from build123d import *

# Parameters (mm, degrees)
CROQUIS1_W              = 164.9
CROQUIS1_H              = 102
SALIENTE_EXTRUIR2_DEPTH = 14.27
CROQUIS2_W              = 174.9
CROQUIS2_H              = 112
CROQUIS2_W_2            = 166.9
CROQUIS2_H_2            = 104
SALIENTE_EXTRUIR3_DEPTH = 14.27
CROQUIS3_W              = 174.9
CROQUIS3_H              = 112
CROQUIS3_W_2            = 160.9
CROQUIS3_H_2            = 98.374406292
SALIENTE_EXTRUIR5_DEPTH = 1
CROQUIS4_W              = 164.9
CROQUIS4_H              = 102
CORTAR_EXTRUIR2_DEPTH   = 14.27
CROQUIS6_W              = 174.9
CROQUIS6_H              = 112
CROQUIS6_R              = 1.5
SALIENTE_EXTRUIR6_DEPTH = 15
CROQUIS8_W              = 160.9
CROQUIS8_H              = 98.374406292
CORTAR_EXTRUIR3_DEPTH   = 9
CROQUIS9_W              = 166.9
CROQUIS9_H              = 104
CORTAR_EXTRUIR5_DEPTH   = 11
CROQUIS15_W             = 6.3
CROQUIS15_H             = 15
CROQUIS15_W_2           = 3.5
CROQUIS15_H_2           = 7
CORTAR_EXTRUIR6_DEPTH   = 7
CORTAR_EXTRUIR7_DEPTH   = 7
CROQUIS17_R             = 4
CORTAR_EXTRUIR8_DEPTH   = 7
CROQUIS18_W             = 4
CROQUIS18_H             = 16
CORTAR_EXTRUIR9_DEPTH   = 7
CROQUIS21_R             = 1.5
CORTAR_EXTRUIR12_DEPTH  = 25.4
CROQUIS22_W             = 4.034105038
CROQUIS22_H             = 112
CORTAR_EXTRUIR13_DEPTH  = 179.4


with BuildPart() as part:
    # Croquis1 → Saliente-Extruir2 (new body)
    with BuildSketch(Plane(origin=(0, 0, 0), x_dir=(0, 0, -1), z_dir=(1, 0, 0))):
        Rectangle(CROQUIS1_W, CROQUIS1_H)
    extrude(amount=SALIENTE_EXTRUIR2_DEPTH)

    # Croquis4 → Cortar-Extruir2 (cut)
    with BuildSketch(Plane(origin=(14.27, 0, 0), x_dir=(0, 0, -1), z_dir=(1, 0, 0))):
        Rectangle(CROQUIS4_W, CROQUIS4_H)
    extrude(amount=-CORTAR_EXTRUIR2_DEPTH, mode=Mode.SUBTRACT)


with BuildPart() as body_2:
    # Croquis2 → Saliente-Extruir3 (new body)
    with BuildSketch(Plane(origin=(0, 0, 0), x_dir=(0, 0, -1), z_dir=(1, 0, 0))):
        Rectangle(CROQUIS2_W, CROQUIS2_H)
        Rectangle(CROQUIS2_W_2, CROQUIS2_H_2, mode=Mode.SUBTRACT)
    extrude(amount=SALIENTE_EXTRUIR3_DEPTH)

    # Croquis3 → Saliente-Extruir5 (add)
    with BuildSketch(Plane.ZY):
        Rectangle(CROQUIS3_W, CROQUIS3_H)
        with Locations((0, -0.062203146)):
            Rectangle(CROQUIS3_W_2, CROQUIS3_H_2, mode=Mode.SUBTRACT)
    extrude(amount=SALIENTE_EXTRUIR5_DEPTH)

    # Croquis6 → Saliente-Extruir6 (add)
    with BuildSketch(Plane(origin=(14.27, 0, 0), x_dir=(0, 0, -1), z_dir=(1, 0, 0))):
        Rectangle(CROQUIS6_W, CROQUIS6_H)
        with Locations((-77.445, 46)):
            Circle(CROQUIS6_R, mode=Mode.SUBTRACT)
        with Locations((-77.445, -46)):
            Circle(CROQUIS6_R, mode=Mode.SUBTRACT)
        with Locations((-22.1, 15.81)):
            Circle(CROQUIS6_R, mode=Mode.SUBTRACT)
        with Locations((35.9, 15.81)):
            Circle(CROQUIS6_R, mode=Mode.SUBTRACT)
        with Locations((-22.1, -33.19)):
            Circle(CROQUIS6_R, mode=Mode.SUBTRACT)
        with Locations((35.9, -33.19)):
            Circle(CROQUIS6_R, mode=Mode.SUBTRACT)
        with Locations((77.445, 46)):
            Circle(CROQUIS6_R, mode=Mode.SUBTRACT)
        with Locations((77.445, -46)):
            Circle(CROQUIS6_R, mode=Mode.SUBTRACT)
    extrude(amount=SALIENTE_EXTRUIR6_DEPTH)

    # Croquis8 → Cortar-Extruir3 (cut)
    with BuildSketch(Plane.ZY.offset(-14.27)):
        with Locations((0, -0.062203146)):
            Rectangle(CROQUIS8_W, CROQUIS8_H)
    extrude(amount=-CORTAR_EXTRUIR3_DEPTH, mode=Mode.SUBTRACT)

    # Croquis9 → Cortar-Extruir5 (cut)
    with BuildSketch(Plane.ZY.offset(-14.27)):
        Rectangle(CROQUIS9_W, CROQUIS9_H)
    extrude(amount=-CORTAR_EXTRUIR5_DEPTH, mode=Mode.SUBTRACT)

    # Croquis15 → Cortar-Extruir6 (cut)
    with BuildSketch(Plane.XY.offset(87.45)):
        with Locations((18.42, 9.417324545)):
            Rectangle(CROQUIS15_W, CROQUIS15_H)
        with Locations((17.02, -11.082675455)):
            Rectangle(CROQUIS15_W_2, CROQUIS15_H_2)
        with Locations((17.02, -29.082675455)):
            Rectangle(CROQUIS15_W_2, CROQUIS15_H_2)
    extrude(amount=-CORTAR_EXTRUIR6_DEPTH, mode=Mode.SUBTRACT)

    # Croquis16 → Cortar-Extruir7 (cut)
    with BuildSketch(Plane(origin=(29.27, 0, 0), x_dir=(0, 0, -1), z_dir=(1, 0, 0))):
        with BuildLine():
            Line((-70.67585332, 19.450942007), (-40.125245351, 19.450942007))
            ThreePointArc((-40.125245351, 19.450942007), (-36.589711445, 20.915408101), (-35.125245351, 24.450942007))
            Line((-35.125245351, 24.450942007), (-35.125245351, 43.370497663))
            ThreePointArc((-35.125245351, 43.370497663), (-36.589711445, 46.906031569), (-40.125245351, 48.370497663))
            Line((-40.125245351, 48.370497663), (-70.67585332, 48.370497663))
            ThreePointArc((-70.67585332, 48.370497663), (-74.211387226, 46.906031569), (-75.67585332, 43.370497663))
            Line((-75.67585332, 43.370497663), (-75.67585332, 24.450942007))
            ThreePointArc((-75.67585332, 24.450942007), (-74.211387226, 20.915408101), (-70.67585332, 19.450942007))
        make_face()
        with BuildLine():
            Line((40.269537366, 19.465768949), (70.820145334, 19.465768949))
            ThreePointArc((70.820145334, 19.465768949), (74.35567924, 20.930235043), (75.820145334, 24.465768949))
            Line((75.820145334, 24.465768949), (75.820145334, 43.385324606))
            ThreePointArc((75.820145334, 43.385324606), (74.35567924, 46.920858512), (70.820145334, 48.385324606))
            Line((70.820145334, 48.385324606), (40.269537366, 48.385324606))
            ThreePointArc((40.269537366, 48.385324606), (36.73400346, 46.920858512), (35.269537366, 43.385324606))
            Line((35.269537366, 43.385324606), (35.269537366, 24.465768949))
            ThreePointArc((35.269537366, 24.465768949), (36.73400346, 20.930235043), (40.269537366, 19.465768949))
        make_face()
    extrude(amount=-CORTAR_EXTRUIR7_DEPTH, mode=Mode.SUBTRACT)

    # Croquis17 → Cortar-Extruir8 (cut)
    with BuildSketch(Plane(origin=(0, 0, -87.45), x_dir=(-1, 0, 0), z_dir=(0, 0, -1))):
        with Locations(Location((-17.79171335, -27.901665979, 0), (0, 0, 90))):
            Circle(CROQUIS17_R)
    extrude(amount=-CORTAR_EXTRUIR8_DEPTH, mode=Mode.SUBTRACT)

    # Croquis18 → Cortar-Extruir9 (cut)
    with BuildSketch(Plane(origin=(0, 0, -87.45), x_dir=(-1, 0, 0), z_dir=(0, 0, -1))):
        with Locations((-17.27, -3.082675455)):
            Rectangle(CROQUIS18_W, CROQUIS18_H)
    extrude(amount=-CORTAR_EXTRUIR9_DEPTH, mode=Mode.SUBTRACT)

    # Croquis21 → Cortar-Extruir12 (cut)
    with BuildSketch(Plane(origin=(29.27, 0, 0), x_dir=(0, 0, -1), z_dir=(1, 0, 0))):
        with Locations((-84.95, 53.5)):
            Circle(CROQUIS21_R)
        with Locations((84.95, 53.5)):
            Circle(CROQUIS21_R)
        with Locations((84.95, -53.5)):
            Circle(CROQUIS21_R)
        with Locations((-84.95, -53.5)):
            Circle(CROQUIS21_R)
    extrude(amount=-CORTAR_EXTRUIR12_DEPTH, mode=Mode.SUBTRACT)

    # Croquis22 → Cortar-Extruir13 (cut)
    with BuildSketch(Plane(origin=(0, 0, -87.45), x_dir=(-1, 0, 0), z_dir=(0, 0, -1))):
        with Locations((-27.252947481, 0)):
            Rectangle(CROQUIS22_W, CROQUIS22_H)
    extrude(amount=-CORTAR_EXTRUIR13_DEPTH, mode=Mode.SUBTRACT)


solid = body_2.part
Could you check a few things on this model? Use its own coordinates, in mm. A direction names the side the tool comes from. Give positions to 0.01 mm unless a question says otherwise; leave off trailing zeros. Write each loop counter-clockwise with the first axis right and the second up, starting at its lowest first coordinate (ties: lowest second). Pieces come first, ordered by that corner, then holes. Notation, with made-up numbers: (72, 70.5) -> (95, 70.5) arc R8 cw to (95, 74.5) -> close; hole circle Ø11 at (-19.75, 17). An arc over 180 degrees is marked (long way). Answer as CSV lines item,"result". Start each with the question number.
(1) I'm going to push flat-ended pins straight in: pin 1 Ø1.8 at (y, z) = (53.5, 84.95) entering from +X; pin 2 Ø3.5 at (y, z) = (53.5, -85) entering from +X; pin 3 Ø10 at (y, z) = (40, 22.5) entering from +X. Where does each tip first touch, or does it pass through?
(2) If we section it at B-B, the plane z = 26.5: Write out the boundary of the cut face in (x, y) (3 decimals), and give its area (3 significant figures).
(3) Which directions (+Z, -Z, +X, -X, +Y, -Y) give clear straight access to the entire face, cutting with the end or side of a thin tool? Please do faces 4 (the face through (12, -52, -1)), 5 (the face through (17, 4.917, -85)), 6 (the face through (15.27, -29, 85)).
(4) If we section it at A-A, the plane y = 38.5: Write out the boundary of the cut face in (x, z), and give its area (3 significant figures).
(5) If we section it at C-C, the plane x = 6.5: Write out the boundary of the cut face in (y, z).
(6) Please list where these lines run through material, in increasing order: line 1 (Y direction, x = 9.5, z = -84.95); line 2 (Y direction, x = 20, z = -26); line 3 (Z direction, x = 5.75, y = -23.5).
(7) If we section it at D-D, the plane y = -28.5: Write out the boundary of the cut face in (x, z), and give its area (3 significant figures).
(8) If we mould it in two halves opening along X, with no side actions, what happens to faces 1 (the face through (18.77, -11, 85)), 2 (the face through (12, -1, -83.45)), 3 (the face through (25.236, -54, -7))? For each: +X half, -X half, draft (parallel to the pull), parting line (faces both ways), or undercut.
Answer list:
1,pin 1,"x = 3.87"
1,pin 2,"x = 25.24"
1,pin 3,"through"
2,outline,"(-1, -56) -> (25.236, -56) -> (25.236, -52) -> (0, -52) -> (0, -49.249) -> (-1, -49.249) -> close; (-1, 49.125) -> (0, 49.125) -> (0, 52) -> (25.236, 52) -> (25.236, 56) -> (-1, 56) -> close"
2,area,"216 mm^2"
3,face 4,"+X"
3,face 5,"+Z, -Z"
3,face 6,"+Z"
4,outline,"(-1, -87.45) -> (25.24, -87.45) -> (25.24, -83.45) -> (0, -83.45) -> (0, -80.45) -> (-1, -80.45) -> close; (-1, 80.45) -> (0, 80.45) -> (0, 83.45) -> (25.24, 83.45) -> (25.24, 87.45) -> (-1, 87.45) -> close"
4,area,"216 mm^2"
5,outline,"(-56, -87.45) -> (56, -87.45) -> (56, 87.45) -> (-56, 87.45) -> close; hole circle Ø3 at (-53.5, -84.95); hole circle Ø3 at (-53.5, 84.95); hole (-52, -83.45) -> (52, -83.45) -> (52, 83.45) -> (-52, 83.45) -> close; hole circle Ø3 at (53.5, -84.95); hole circle Ø3 at (53.5, 84.95)"
6,line 1,"-56 to -55, -52 to 52, 55 to 56"
6,line 2,"-56 to -52, 52 to 56"
6,line 3,"-87.45 to -83.45, 83.45 to 87.45"
7,outline,"(-1, -87.45) -> (13.84, -87.45) -> (13.84, -83.45) -> (0, -83.45) -> (0, -80.45) -> (-1, -80.45) -> close; (-1, 80.45) -> (0, 80.45) -> (0, 83.45) -> (15.27, 83.45) -> (15.27, 87.45) -> (-1, 87.45) -> close; (18.77, 83.45) -> (25.24, 83.45) -> (25.24, 87.45) -> (18.77, 87.45) -> close; (21.75, -87.45) -> (25.24, -87.45) -> (25.24, -83.45) -> (21.75, -83.45) -> close"
7,area,"170 mm^2"
8,face 1,"undercut"
8,face 2,"draft"
8,face 3,"+X half"
